Geometry check sheet. Reference: the model listing, model coordinates, mm. Round coordinates to 2 decimals unless told otherwise and drop trailing zeros. Write each loop counter-clockwise with the first axis right and the second up, starting at its lowest first coordinate (ties: lowest second). Pieces come first, ordered by that corner, then holes. Notation, with made-up numbers: (-27.5, 20) - (-7.5, 20) arc R26 ccw to (-7.5, 57) - close; hole circle Ø11 at (40, -15). An arc over 180 degrees is marked (long way). Return JSON: item names as keys, results as strings. Group by question number.
from build123d import *

# Parameters (mm, degrees)
F1_DEPTH    = 5.08
F2_T1_DEPTH = 107.0243637673
F3_SIZE     = 5.07999


# Not quite as in the source:
# - a fillet or chamfer that OpenCascade refuses, or shapes differently, is made with other operations: its cross-section is extruded or revolved along the edge and cut away or added
# - a fillet or chamfer is up to 0.001 mm smaller than in the source, because OpenCascade refuses the exact size


with BuildPart() as f1:
    # F0 (on Top) → F1 (new body)
    with BuildSketch(Plane.XY):
        Polygon((0, 36.2825095654), (0, 0), (52.3514412344, 62.6247823238), (52.3514412344, 79.496473074), align=None)
    extrude(amount=F1_DEPTH)

    # F2: fillet of radius 5.08 on 2 edges, made by hand

    # F2_s2 → F2_t1 (cut)
    with BuildSketch(Plane(origin=(-8.1454025856, -9.7438399371, 0), x_dir=(0, 0, 1), z_dir=(0.6413702823, 0.7672314911, 0))):
        with BuildLine():
            ThreePointArc((0, 0), (3.5921024484, -1.4878975516), (5.08, -5.08))
            Line((5.08, -5.08), (5.08, 0))
            Line((5.08, 0), (0, 0))
        make_face()
        with BuildLine():
            ThreePointArc((5.08, 0), (1.4878975516, -1.4878975516), (0, -5.08))
            Line((0, -5.08), (0, 0))
            Line((0, 0), (5.08, 0))
        make_face()
    extrude(amount=F2_T1_DEPTH, mode=Mode.SUBTRACT)

    # F3 (size 5.08 in the source; OpenCascade refuses exactly that, so slightly less here)
    f3_edges = [f1.edges().sort_by_distance(p)[0] for p in [
        (26.175721, 57.889491, 5.08),
    ]]
    chamfer(f3_edges, length=F3_SIZE)


solid = f1.part
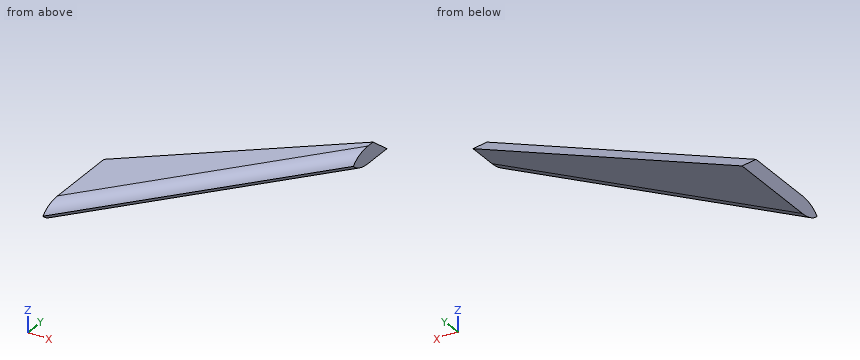
1. Depth check by flat-ended pin: pin 1 Ø4 at (x, y) = (32.5, 62.5) entering from -Z; pin 2 Ø2 at (y, z) = (68, 1.5) entering from -X; pin 3 Ø2 at (x, z) = (38, 4) entering from -Y; pin 4 Ø6 at (x, y) = (30, 60) entering from +Z. Enter the tip coordinate at first touch or a pass-through.
2. Section check A-A (z = 3.4). Enter the section's corners in (x, y), and give its area (3 significant figures).
3. Material ranges on line 1 along Z through (x, y) = (23, 52); line 2 along Y through (x, z) = (4.5, 1); line 3 along X through (y, z) = (62, 3.25), recorded low to high.
Result sheet:
{
 "1": {"pin 1": "stops at z = 0", "pin 2": "stops at x = 38.8", "pin 3": "stops at y = 46.5", "pin 4": "stops at z = 3.81"},
 "2": {"outline": "(0, 2.04) - (52.35, 64.66) - (52.35, 75.09) - (0, 31.87) - close", "area": "1,050 mm²"},
 "3": {"line 1": "z = 0 to 2.52", "line 2": "y = 8.58 to 38.7", "line 3": "x = 36.26 to 50.3"}
}
